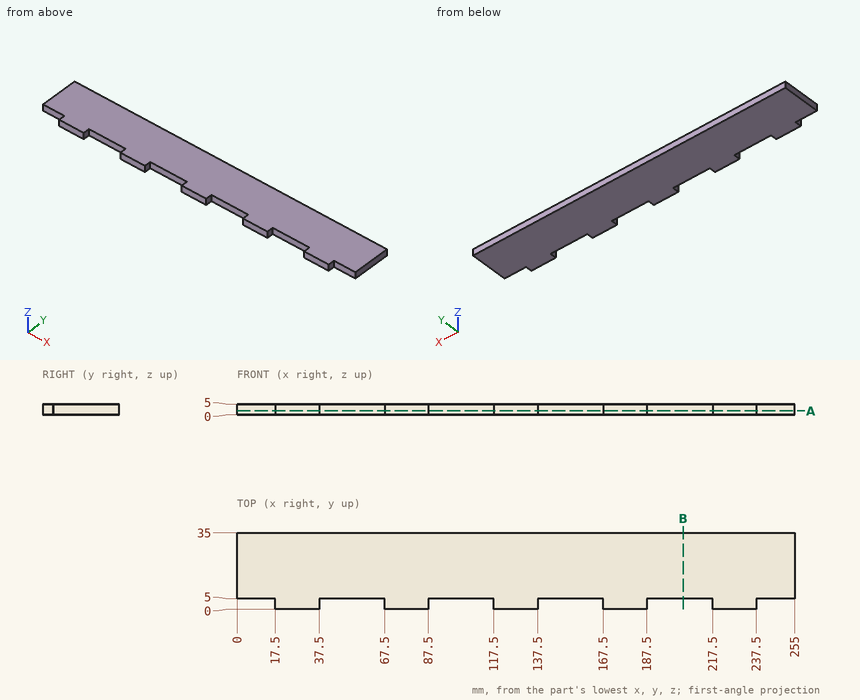
Print and shaded views of the part. All mm, measured from the part's lowest x, y and z. Coordinates: 2 decimals unless noted, no trailing zeros. Order: outer loops, then holes, each group sorted by start corner. A loop starts at its lowest first (then second) coordinate and runs counter-clockwise, first axis right, second up. Notation, with made-up numbers: (-6.75, 6) - (21.25, 6) arc R23 cw to (21.25, 15) - close; hole circle Ø10 at (5, 87.25). An arc over 180 degrees is marked (long way). Put each result on its own line as item: value.
1. Probe line 1 along X through (y, z) = (3.5, 4.85); line 2 along Y through (x, z) = (167, 4.65). List the from-to ranges inside material, lowest first. Write a range as [from, to].
Answer sheet:
line 1: x = [17.5, 37.5], [67.5, 87.5], [117.5, 137.5], [167.5, 187.5], [217.5, 237.5]
line 2: y = [5, 35]
2. Saw through at A-A (z = 1.9). Write the cut outline in (x, y), and give its area (3 significant figures).
Answer sheet:
outline: (0, 5) - (17.5, 5) - (17.5, 0) - (37.5, 0) - (37.5, 5) - (67.5, 5) - (67.5, 0) - (87.5, 0) - (87.5, 5) - (117.5, 5) - (117.5, 0) - (137.5, 0) - (137.5, 5) - (167.5, 5) - (167.5, 0) - (187.5, 0) - (187.5, 5) - (217.5, 5) - (217.5, 0) - (237.5, 0) - (237.5, 5) - (255, 5) - (255, 35) - (0, 35) - close
area: 8,150 mm^2
3. Drop flat-ended pins along their axis: P1, Ø1.5, axis at y = 3.5, z = 3, coming from the -X side; P2, Ø2.5, axis at x = 6, z = 3.5, coming from the -Y side; P3, Ø1.5, axis at y = 2, z = 1.5, coming from the +X side. Give the stop position or say it passes through.
Answer sheet:
P1: stops at x = 17.5
P2: stops at y = 5
P3: stops at x = 237.5
4. Saw through at B-B (x = 204). Write the cut outline in (y, z), and give its area (3 significant figures).
Answer sheet:
outline: (5, 0) - (35, 0) - (35, 5) - (5, 5) - close
area: 150 mm^2
